```python
from build123d import *

# Parameters (mm, degrees)
F0_R      = 7
F1_DEPTH  = 2
F2_R      = 9
F3_DEPTH  = 2
F3_FACE_R = 9
F5_R      = 2.5


with BuildPart() as f1:
    # F0 (on Top) → F1 (new body)
    with BuildSketch(Plane.XY):
        Circle(F0_R)
    extrude(amount=F1_DEPTH)

    # F2 (on face) → F3 (join)
    with BuildSketch(Plane.XY.offset(2)):
        Circle(F2_R)
    extrude(amount=F3_DEPTH)

    # F3_face (on face) → F6 section 0
    with BuildSketch(Plane.XY.offset(4)):
        Circle(F3_FACE_R)
    # F5 (on offset) → F6 section 1
    with BuildSketch(Plane.XY.offset(29)):
        Circle(F5_R)
    loft()

    # F7 (on face) → F8 (revolve)
    with BuildSketch(Plane.XY.offset(29)):
        with BuildLine():
            Line((-2.5, 0), (2.5, 0))
            ThreePointArc((2.5, 0), (0, 2.5), (-2.5, 0))
        make_face()
        with BuildLine():
            ThreePointArc((-5, 0), (0, -5), (5, 0))
            Line((5, 0), (2.5, 0))
            ThreePointArc((2.5, 0), (0, -2.5), (-2.5, 0))
            Line((-2.5, 0), (-5, 0))
        make_face()
    revolve(axis=Axis((0, 0, 29), (1, 0, 0)))


solid = f1.part
```
Here's how the part is built. I have some questions about the finished solid (model axes, mm). A direction names the side the tool comes from. Round coordinates to 2 decimals unless told otherwise and drop trailing zeros. Write each loop counter-clockwise with the first axis right and the second up, starting at its lowest first coordinate (ties: lowest second). Pieces come first, ordered by that corner, then holes. Notation, with made-up numbers: M 77,-8 L 127,-8 A24 cw 127,16 Z; hole C 25,89 d3. An arc over 180 degrees is marked long. Answer as CSV lines item,"result". Start each with the question number.
1. On a 3-axis mill with a long thin cutter (end or side, diameter ignored), from which of +Z, -Z, +X, -X, +Y, -Y can I reach the whole of each face in a straight line? I mean faces 1 (the conical face through (-1.206, -5.433, 17.212)), 2 (the cylindrical face through (-1.172, 8.923, 2.986)), 3 (the flat face through (0, -7.3, 2)). Say none if no direction works.
2. Suppose I cut it at B-B on x = 0. Write out the boundary of the cut face in (y, z).
3. I'm going to push flat-ended pins straight in: pin 1 Ø5 at (x, z) = (4, 14.5) entering from +Y; pin 2 Ø2 at (x, y) = (0.5, 6) entering from -Z; pin 3 Ø2 at (x, y) = (-2, -4) entering from +Z; pin 4 Ø2 at (y, z) = (0, 12) entering from -X. Where does each tip first touch, or does it pass through?
4. Suppose I cut it at C-C on z = 9. Write out the boundary of the cut face in (x, y).
5. Suppose I cut it at A-A on z = 18.5. Write out the boundary of the cut face in (x, y).
6. I need wall thicknesses on probe 1 along Y at (x, z) = (-1.5, 12); probe 2 along X at (y, z) = (4.5, 11); probe 3 along Y at (x, z) = (-3, 31). Which ranges of each line are inside material? Lowest first, please.
Check result:
1,face 1,"none"
1,face 2,"+Z, -Z"
1,face 3,"-Z"
2,outline,"M -9,2 L -7,2 L -7,0 L 7,0 L 7,2 L 9,2 L 9,4 L 3.44,25.37 A5 ccw long -3.44,25.37 L -9,4 Z"
3,pin 1,"stops at y = 6.35"
3,pin 2,"stops at z = 0"
3,pin 3,"stops at z = 32.6"
3,pin 4,"stops at x = -7.18"
4,outline,"C 0,0 d15.4"
5,outline,"C 0,0 d10.46"
6,probe 1,"y = -6.76 to 6.76"
6,probe 2,"x = -5.59 to 5.59"
6,probe 3,"y = -3.46 to 3.46"
